Source: CAD feature listing. Evaluate the final solid. Frame: model axes, mm. A direction names the side the tool comes from. Coordinates: 2 decimals unless noted, no trailing zeros. Order: outer loops, then holes, each group sorted by start corner. A loop starts at its lowest first (then second) coordinate and runs counter-clockwise, first axis right, second up. Notation, with made-up numbers: (18.5, 16) - (56.5, 16) arc R31 cw to (56.5, 46) - close; hole circle Ø10 at (-39, 12.25). An arc over 180 degrees is marked (long way). One line per question, with ' | ' between items.
from build123d import *

# Parameters (mm, degrees)
SKETCH1_W           = 30
SKETCH1_H           = 52
BOSS_EXTRUDE1_DEPTH = 20
SKETCH3_W           = 15
SKETCH3_H           = 6.1
CUT_EXTRUDE1_DEPTH  = 69.886771008
SKETCH4_R           = 2.5
BOSS_EXTRUDE2_DEPTH = 40


with BuildPart() as part:
    # Sketch1 → Boss-Extrude1 (new body)
    with BuildSketch(Plane.XY):
        with Locations((25.514037319, -26)):
            Rectangle(SKETCH1_W, SKETCH1_H)
    extrude(amount=BOSS_EXTRUDE1_DEPTH)

    # Sketch3 → Cut-Extrude1 (cut, through all)
    with BuildSketch(Plane(origin=(0, 0, 0), x_dir=(1, 0, 0), z_dir=(0, 1, 0))):
        with Locations((18.014037319, -9.05)):
            Rectangle(SKETCH3_W, SKETCH3_H)
    extrude(amount=-CUT_EXTRUDE1_DEPTH, mode=Mode.SUBTRACT)

    # Sketch4 → Boss-Extrude2 (add)
    with BuildSketch(Plane(origin=(0, -52, 0), x_dir=(-1, 0, 0), z_dir=(0, -1, 0))):
        with Locations((-31.514037319, -9.05)):
            Circle(SKETCH4_R)
    extrude(amount=BOSS_EXTRUDE2_DEPTH)


solid = part.part
(1) Material intervals for L1, parallel to Z at x = 13.5, y = -7; L2, parallel to Y at x = 21.5, z = 3.25; L3, parallel to X at y = -9, z = 8, sorted ascending. Write a range as from..to.
Taken from the geometry:
L1: z = 0..6, 12.1..20 | L2: y = -52..0 | L3: x = 25.51..40.51
(2) Cut plane C-C (y = -22). Return the cut outline in (x, z).
Taken from the geometry:
outline: (10.51, 0) - (40.51, 0) - (40.51, 20) - (10.51, 20) - (10.51, 12.1) - (25.51, 12.1) - (25.51, 6) - (10.51, 6) - close
(3) Cut plane B-B (z = 9.05). Return the cut outline in (x, y).
Taken from the geometry:
outline: (25.51, -52) - (29.01, -52) - (29.01, -92) - (34.01, -92) - (34.01, -52) - (40.51, -52) - (40.51, 0) - (25.51, 0) - close
(4) Set-up query: faces 5 (the flat face through (25.514, -26, 9)), 6 (the flat face through (10.514, -26, 3)). Return all of +Z, -Z, +X, -X, +Y, -Y with unobstructed straight access to the full face (end or side cutting, diameter ignored); none if empty.
Taken from the geometry:
face 5: -X, +Y, -Y | face 6: +Z, -Z, -X, +Y, -Y
(5) Cut plane A-A (x = 18). Return the cut outline in (y, z), and give its area (3 significant figures).
Taken from the geometry:
outline: (-52, 0) - (0, 0) - (0, 6) - (-52, 6) - close; (-52, 12.1) - (0, 12.1) - (0, 20) - (-52, 20) - close | area: 723 mm²
(6) Pull-direction query (Z, two-part tool) for faces 1 (the flat face through (18, -26, 12.1)), 2 (the cylindrical face through (34.01, -71.72, 8.94)), 3 (the flat face through (18, -26, 6)), 4 (the flat face through (32, -92, 9)); classes: pulls with the +Z half, pulls with the -Z half, needs draft (parallel to the pull), parting line crosses it, or undercut.
Taken from the geometry:
face 1: undercut | face 2: parting line crosses it | face 3: undercut | face 4: needs draft
(7) Pin query (flat end, axial travel): P1, Ø1.5, axis at x = 32.5, z = 3.5, coming from the -Y side; P2, Ø6, axis at x = 31, z = 13.5, coming from the -Y side. Return the tip coordinate at first contact, or that it passes through.
Taken from the geometry:
P1: stops at y = -52 | P2: stops at y = -92
(8) Cut plane D-D (x = 38). Return the cut outline in (y, z).
Taken from the geometry:
outline: (-52, 0) - (0, 0) - (0, 20) - (-52, 20) - close
